The listing builds one solid part. Answer for the finished solid, in the listing's coordinates (mm). Face numbers are marked on the shaded views. A direction names the side the tool comes from. Coordinates: 2 decimals unless noted, no trailing zeros. Loops run counter-clockwise (first coordinate to the right, second up) from the corner with the lowest first, then second, coordinate; pieces in that order, holes last. Notation, with made-up numbers: M 46,22.25 L 65,22.25 A27 ccw 65,51.25 Z; hole C -0.75,-13 d3. An arc over 180 degrees is marked long. Return JSON: item names as keys, results as strings. Group by question number.
1. Section A-A (x = 0) is taken. Write down the section's boundary in (y, z), then the cut area to 3 significant figures.
2. Given P1, Ø1.1, axis at x = 17.5, z = -8.5, coming from the +Y side; P2, Ø4, axis at x = -16.5, y = 17, coming from the -Z side; P3, Ø1.4, axis at x = 16.5, y = 17.5, coming from the +Z side, each flat-ended and moving along its own axis, determine where each tip first touches the part or whether it passes through.
3. Which of the six approach directions +Z, -Z, +X, -X, +Y, -Y give full straight-line access (tool end or side, diameter ignored) to the marked faces 4, 5 and 6?
4. Straight lines are drawn through the part: L1, parallel to X at y = -17, z = -4.75; L2, parallel to X at y = 14, z = -6. For each, find the intervals that lie inside material, in ascending order. Write a range as from..to.
5. Section B-B (y = 9) is taken. Write down the section's boundary in (x, z).
6. Section D-D (z = -7.6) is taken. Count the separate pieces of the cut face and the enclosed holes in it, then the cut area to 3 significant figures.
7. The mould has two halves that part along Z. Classify the marked faces 1, 2 and 3: pulls with the +Z half, pulls with the -Z half, needs draft (parallel to the pull), parting line crosses it, or undercut.
```python
from build123d import *

# Parameters (mm, degrees)
SKETCH1_W           = 42.5
SKETCH1_H           = 42.5
SKETCH1_W_2         = 38.5
SKETCH1_H_2         = 38.5
BOSS_EXTRUDE2_DEPTH = 15.2
SKETCH2_R           = 1.2
BOSS_EXTRUDE4_DEPTH = 11.6
BOSS_EXTRUDE5_DEPTH = 15.2
CIRPATTERN1_COUNT   = 4
CUT_EXTRUDE2_DEPTH  = 4
CUT_EXTRUDE3_REACH  = 58.315
SKETCH4_R           = 3.5
FILLET1_R           = 2


with BuildPart() as part:
    # Sketch1 → Boss-Extrude2 (new body)
    with BuildSketch(Plane.XY):
        Rectangle(SKETCH1_W, SKETCH1_H)
        Rectangle(SKETCH1_W_2, SKETCH1_H_2, mode=Mode.SUBTRACT)
    extrude(amount=-BOSS_EXTRUDE2_DEPTH)

    # Sketch2 → Boss-Extrude4 (add)
    # profile 1 of 4: a face of its own
    with BuildSketch(Plane(origin=(0, 0, -1.6), x_dir=(-1, 0, 0), z_dir=(0, 0, -1))):
        with BuildLine():
            Line((17, -14.55), (19.25, -14.55))
            Line((19.25, -14.55), (19.25, -19.25))
            Line((19.25, -19.25), (14.55, -19.25))
            Line((14.55, -19.25), (14.55, -17))
            ThreePointArc((14.55, -17), (15.267588386, -15.267588386), (17, -14.55))
        make_face()
        with Locations(Location((17, -17, 0), (0, 0, 90))):
            Circle(SKETCH2_R, mode=Mode.SUBTRACT)
    # profile 2 of 4: a face of its own
    with BuildSketch(Plane(origin=(0, 0, -1.6), x_dir=(-1, 0, 0), z_dir=(0, 0, -1))):
        with BuildLine():
            Line((19.25, 14.55), (19.25, 19.25))
            Line((19.25, 19.25), (14.55, 19.25))
            Line((14.55, 19.25), (14.55, 17))
            ThreePointArc((14.55, 17), (15.267588386, 15.267588386), (17, 14.55))
            Line((17, 14.55), (19.25, 14.55))
        make_face()
        with Locations(Location((17, 17, 0), (0, 0, 180))):
            Circle(SKETCH2_R, mode=Mode.SUBTRACT)
    # profile 3 of 4: a face of its own
    with BuildSketch(Plane(origin=(0, 0, -1.6), x_dir=(-1, 0, 0), z_dir=(0, 0, -1))):
        with BuildLine():
            Line((-19.25, -14.55), (-19.25, -19.25))
            Line((-19.25, -19.25), (-14.55, -19.25))
            Line((-14.55, -19.25), (-14.55, -17))
            ThreePointArc((-14.55, -17), (-15.267588386, -15.267588386), (-17, -14.55))
            Line((-17, -14.55), (-19.25, -14.55))
        make_face()
        with Locations(Location((-17, -17, 0), (0, 0, 180))):
            Circle(SKETCH2_R, mode=Mode.SUBTRACT)
    # profile 4 of 4: a face of its own
    with BuildSketch(Plane(origin=(0, 0, -1.6), x_dir=(-1, 0, 0), z_dir=(0, 0, -1))):
        with BuildLine():
            Line((-17, 14.55), (-19.25, 14.55))
            Line((-19.25, 14.55), (-19.25, 19.25))
            Line((-19.25, 19.25), (-14.55, 19.25))
            Line((-14.55, 19.25), (-14.55, 17))
            ThreePointArc((-14.55, 17), (-15.267588386, 15.267588386), (-17, 14.55))
        make_face()
        with Locations(Location((-17, 17, 0), (0, 0, 90))):
            Circle(SKETCH2_R, mode=Mode.SUBTRACT)
    extrude(amount=BOSS_EXTRUDE4_DEPTH)

    # Sketch5 → Boss-Extrude5 (add)
    with BuildSketch(Plane.XY):
        Polygon((-21.25, 5), (-21.25, -5), (-24.25, -8), (-24.25, 8), align=None)
    boss_extrude5 = extrude(amount=-BOSS_EXTRUDE5_DEPTH)

    # CirPattern1: Boss-Extrude5 ×4 about axis
    cirpattern1_axis = Axis((0, 0, 0), (0, 0, 1))
    for i in range(1, CIRPATTERN1_COUNT):
        add(boss_extrude5.rotate(cirpattern1_axis, i * 360 / CIRPATTERN1_COUNT))

    # Sketch3 → Cut-Extrude2 (cut)
    with BuildSketch(Plane.XY):
        with BuildLine():
            Line((20.25, -11.05), (20.25, -9.55))
            ThreePointArc((20.25, -9.55), (19.542893219, -9.257106781), (19.25, -8.55))
            Line((19.25, -8.55), (19.25, -12.05))
            ThreePointArc((19.25, -12.05), (19.542893219, -11.342893219), (20.25, -11.05))
        make_face()
    extrude(amount=-CUT_EXTRUDE2_DEPTH, mode=Mode.SUBTRACT)

    # Sketch4 → Cut-Extrude3 (cut, up to next)
    with BuildSketch(Plane(origin=(0, 24.25, 0), x_dir=(1, 0, 0), z_dir=(0, 1, 0)), mode=Mode.PRIVATE) as cut_extrude3_sk1:
        with Locations(Location((0, 7.6, 0), (0, 0, 180))):
            Circle(SKETCH4_R)
    cut_extrude3_tool1 = extrude(cut_extrude3_sk1.sketch, amount=-CUT_EXTRUDE3_REACH, mode=Mode.PRIVATE) & part.part
    add(cut_extrude3_tool1.solids().sort_by_distance((0, 24.25, -7.6))[0], mode=Mode.SUBTRACT)

    # Fillet1
    fillet1_edges = [part.edges().sort_by_distance(p)[0] for p in [
        (-21.25, -21.25, -7.6),
        (-21.25, 21.25, -7.6),
        (21.25, 21.25, -7.6),
        (21.25, -21.25, -7.6),
    ]]
    fillet(fillet1_edges, radius=FILLET1_R)


solid = part.part
```
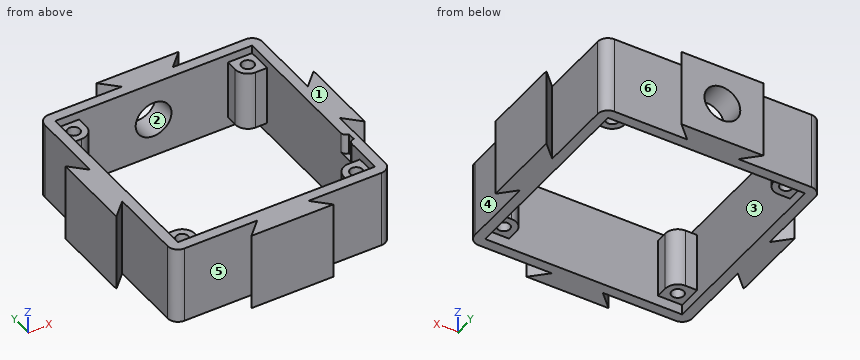
Worked out:
{
 "1": {"outline": "M -24.25,-15.2 L -19.25,-15.2 L -19.25,0 L -24.25,0 Z; M 19.25,-15.2 L 24.25,-15.2 L 24.25,-11.1 L 19.25,-11.1 Z; M 19.25,-4.1 L 24.25,-4.1 L 24.25,0 L 19.25,0 Z", "area": "117 mm^2"},
 "2": {"P1": "y = 21.25", "P2": "z = -13.2", "P3": "z = -1.6"},
 "3": {"face 4": "+Z, -Z, -Y", "face 5": "+Z, -Z, -X", "face 6": "+Z, -Z, +X"},
 "4": {"L1": "-21.25..-18.2, -15.8..-14.55, 14.55..15.8, 18.2..21.25", "L2": "-21.25..-19.25, 19.25..21.25"},
 "5": {"outline": "M -21.25,-15.2 L -19.25,-15.2 L -19.25,0 L -21.25,0 Z; M 19.25,-15.2 L 21.25,-15.2 L 21.25,0 L 19.25,0 Z"},
 "6": {"separate pieces": "1", "enclosed holes": "4", "area": "507 mm^2"},
 "7": {"face 1": "pulls with the +Z half", "face 2": "undercut", "face 3": "needs draft"}
}
